from build123d import *

# Parameters (mm, degrees)
ESQUISSE1_W             = 32
ESQUISSE1_H             = 6
BOSS_EXTRU_1_DEPTH      = 6
ESQUISSE2_R             = 0.625
ENL_V_MAT_EXTRU_1_DEPTH = 34.105890714
ESQUISSE3_R             = 0.625
ENL_V_MAT_EXTRU_2_DEPTH = 34.105890714


with BuildPart() as part:
    # Esquisse1 → Boss.-Extru.1 (new body)
    with BuildSketch(Plane.XY):
        with Locations((-16, -3)):
            Rectangle(ESQUISSE1_W, ESQUISSE1_H)
    extrude(amount=BOSS_EXTRU_1_DEPTH)

    # Esquisse2 → Enlèv. mat.-Extru.1 (cut, through all)
    with BuildSketch(Plane.ZY.offset(32)):
        with Locations((3, -3)):
            Circle(ESQUISSE2_R)
    extrude(amount=-ENL_V_MAT_EXTRU_1_DEPTH, mode=Mode.SUBTRACT)

    # Esquisse3 → Enlèv. mat.-Extru.2 (cut, through all)
    with BuildSketch(Plane.XZ.offset(6)):
        with Locations((-29.5, 3)):
            Circle(ESQUISSE3_R)
        with Locations((-2.5, 3)):
            Circle(ESQUISSE3_R)
    extrude(amount=-ENL_V_MAT_EXTRU_2_DEPTH, mode=Mode.SUBTRACT)


solid = part.part
CAD build for the part. Positions are in the model's coordinates, mm. Coordinates: 2 decimals unless noted, no trailing zeros. Order: outer loops, then holes, each group sorted by start corner. A loop starts at its lowest first (then second) coordinate and runs counter-clockwise, first axis right, second up.
Item 1: Drill centre lines: L1, parallel to X at y = -1.3, z = 3 (3 decimals); L2, parallel to Y at x = -31.4, z = 3 (3 decimals); L3, parallel to Z at x = -29.5, y = -1.85 (3 decimals). Where is each one in solid material? Low to high.
Check sheet entries:
L1: x = -32 to -30.125, -28.875 to -3.125, -1.875 to 0
L2: y = -6 to -3.625, -2.375 to 0
L3: z = 0 to 2.375, 3.625 to 6
Item 2: Two-plate mould, pull along X, no slides. Class faces 1 (the face through (-30.124, -4.854, 3.027)), 2 (the face through (-32, -3, 2)), 3 (the face through (-16, -6, 3)): +X half, -X half, draft (parallel to the pull), parting line (faces both ways), or undercut.
Check sheet entries:
face 1: undercut
face 2: -X half
face 3: draft
Item 3: Band-saw the part on B-B on x = -16.5. List the corners of the cut face in (y, z) (3 decimals), plus the area to 3 significant figures.
Check sheet entries:
outline: (-6, 0) - (0, 0) - (0, 6) - (-6, 6) - close; hole circle Ø1.25 at (-3, 3)
area: 34.8 mm2
Item 4: Band-saw the part on A-A on z = 3. List the corners of the cut face in (x, y) (3 decimals), plus the area to 3 significant figures.
Check sheet entries:
outline: (-32, -6) - (-30.125, -6) - (-30.125, -3.625) - (-32, -3.625) - close; (-32, -2.375) - (-30.125, -2.375) - (-30.125, 0) - (-32, 0) - close; (-28.875, -6) - (-3.125, -6) - (-3.125, -3.625) - (-28.875, -3.625) - close; (-28.875, -2.375) - (-3.125, -2.375) - (-3.125, 0) - (-28.875, 0) - close; (-1.875, -6) - (0, -6) - (0, -3.625) - (-1.875, -3.625) - close; (-1.875, -2.375) - (0, -2.375) - (0, 0) - (-1.875, 0) - close
area: 140 mm2
